Check sheet for the drawn part. Datum: minimum x, y, z corner. Units: mm. Round coordinates to 2 decimals unless told otherwise and drop trailing zeros. Write each loop counter-clockwise with the first axis right and the second up, starting at its lowest first coordinate (ties: lowest second). Pieces come first, ordered by that corner, then holes.
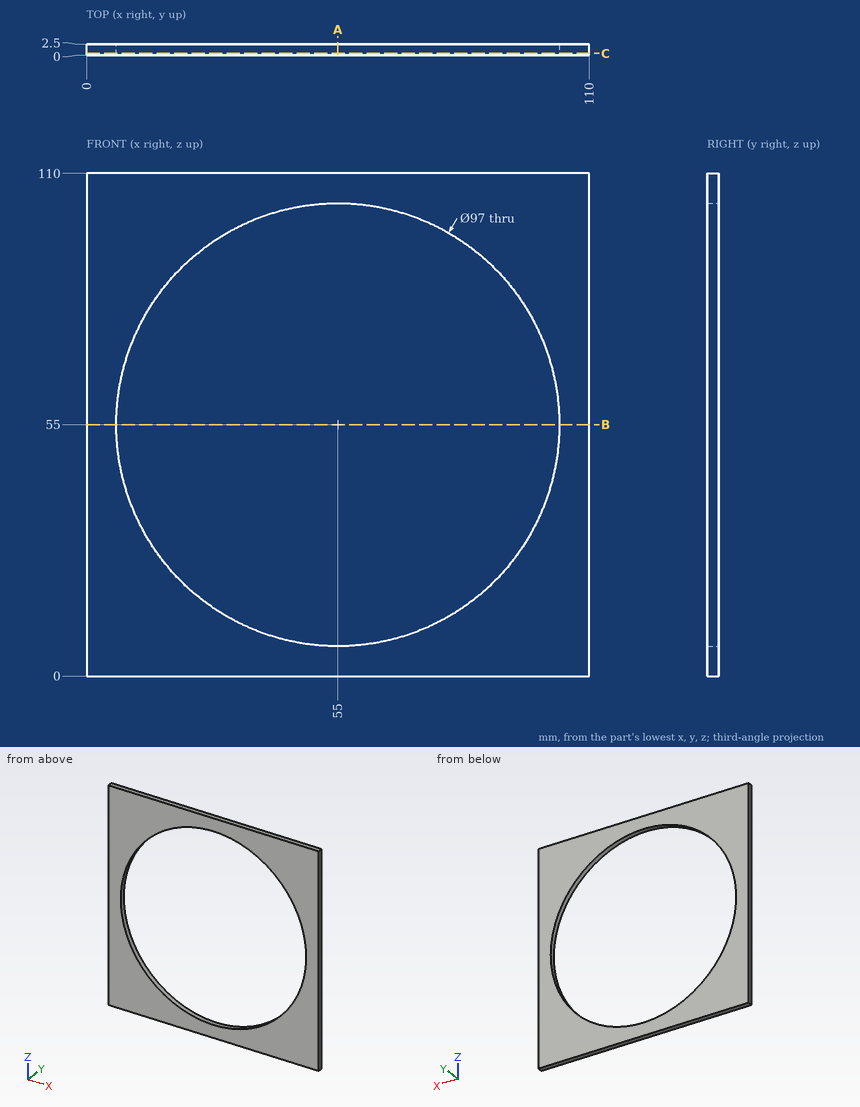
1. Sectioned sample at B-B, the plane z = 55. Enter the section's corners in (x, y).
2. Go/stop test with a flat-tipped pin: pin 1 (12 mm diameter, centred on x = 74.5, z = 11, fed in from +Y). Record where the tip stops, or that it passes through.
3. Sectioned sample at C-C, the plane y = 0.45. Enter the section's corners in (x, z).
4. Sectioned sample at A-A, the plane x = 55. Enter the section's corners in (y, z), plus the area to 3 significant figures.
5. Scan lines: line 1 along Z through (x, y) = (55, 1.35); line 2 along Z through (x, y) = (23, 1.65). Record each from-to range of solid material in increasing order.
Computed values:
1. outline: (0, 0) - (6.5, 0) - (6.5, 2.5) - (0, 2.5) - close; (103.5, 0) - (110, 0) - (110, 2.5) - (103.5, 2.5) - close
2. pin 1: stops at y = 2.5
3. outline: (0, 0) - (110, 0) - (110, 110) - (0, 110) - close; hole circle Ø97 at (55, 55)
4. outline: (0, 0) - (2.5, 0) - (2.5, 6.5) - (0, 6.5) - close; (0, 103.5) - (2.5, 103.5) - (2.5, 110) - (0, 110) - close
4. area: 32.5 mm2
5. line 1: z = 0 to 6.5, 103.5 to 110
5. line 2: z = 0 to 18.55, 91.45 to 110
